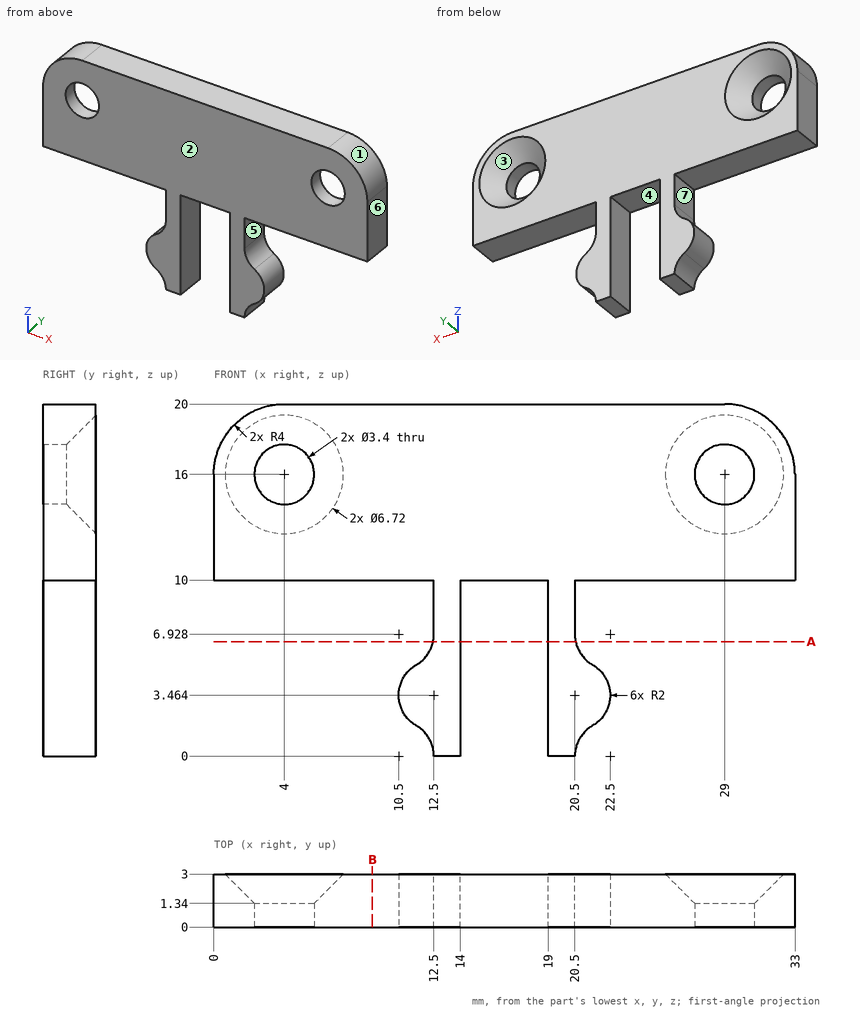
Drawing for the job (mm, zero at the part's lowest x, y, z). A direction names the side the tool comes from. Round coordinates to 2 decimals unless told otherwise and drop trailing zeros. Loops run counter-clockwise (first coordinate to the right, second up) from the corner with the lowest first, then second, coordinate; pieces in that order, holes last. Notation, with made-up numbers: (29.25, -1.75) -> (69.25, -1.75) arc R28 ccw to (69.25, 18.25) -> close; hole circle Ø9 at (65, 62). An arc over 180 degrees is marked (long way). Use one line per item in the form item = value. Start each with the question number.
Item 1: Tool access for the marked faces 4, 5, 6 and 7: list every direction of +Z, -Z, +X, -X, +Y, -Y with a clear straight run to the whole face (end or side of a thin tool).
Item 2: Drop flat-ended pins along their axis: pin 1 Ø1 at (y, z) = (1.5, 16) entering from -X; pin 2 Ø0.9 at (x, y) = (6, 1) entering from -Z; pin 3 Ø1.5 at (y, z) = (1.5, 9) entering from +X. Give the stop position or say it passes through.
Item 3: Band-saw the part on B-B (x = 9). List the corners of the cut face in (y, z).
Item 4: Two-plate mould, pull along Z, no slides. Class the marked faces 1, 2 and 3: released by +Z, released by -Z, zero draft, split by the parting line, or undercut.
Item 5: Drill centre lines: line 1 along X through (y, z) = (0.85, 16); line 2 along Z through (x, y) = (4, 0.8); line 3 along X through (y, z) = (2.8, 18) (1 decimal). Where is each one in solid material? Low to high.
Item 6: Band-saw the part on A-A (z = 6.5). List the corners of the cut face in (x, y).
Data:
q1.face_4 = -Z, +Y, -Y
q1.face_5 = +X, +Y, -Y
q1.face_6 = +Z, -Z, +X, +Y, -Y
q1.face_7 = -X, +Y, -Y
q2.pin_1 = 0
q2.pin_2 = 10
q2.pin_3 = 20.5
q3.outline = (0, 10) -> (3, 10) -> (3, 20) -> (0, 20) -> close
q4.face_1 = released by +Z
q4.face_2 = zero draft
q4.face_3 = undercut
q5.line_1 = 0 to 2.3, 5.7 to 27.3, 30.7 to 33
q5.line_2 = 10 to 14.3, 17.7 to 20
q5.line_3 = 0.5 to 1.6, 6.4 to 26.6, 31.4 to 32.5
q6.outline = (12.45, 0) -> (14, 0) -> (14, 3) -> (12.45, 3) -> close; (19, 0) -> (20.55, 0) -> (20.55, 3) -> (19, 3) -> close
